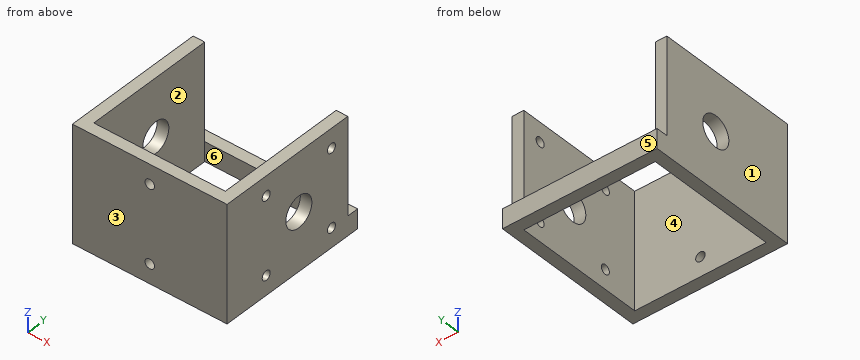
Autodesk Inventor part; units mm, degrees
ref_plane "YZ Plane" through (0, 0, 0) normal (1, 0, 0) x (0, 1, 0)
ref_plane "XZ Plane" through (0, 0, 0) normal (0, 1, 0) x (-1, 0, 0)
ref_plane "XY Plane" through (0, 0, 0) normal (0, 0, 1) x (1, 0, 0)
sketch "スケッチ1" plane through (0, 0, 0) normal (0, 0, 1) x (1, 0, 0)
  line L0 (0, 0) -> (40, 0)
  line L1 (40, 0) -> (40, 40)
  line L2 (40, 40) -> (0, 40)
  line L3 (0, 40) -> (0, 0)
  dimension "d0" = 40
  dimension "d1" = 40
extrude "押し出し1" add sketch "スケッチ1" along normal blind 40
sketch "スケッチ2" plane through (0, 0, 0) normal (0, 0, -1) x (-1, 0, 0)
  point P0 (0, 0)
sketch "スケッチ3" plane through (0, 0, 40) normal (0, 0, 1) x (1, 0, 0)
  line L0 (3, 3) -> (37, 3)
  line L1 (37, 3) -> (37, 37)
  line L2 (37, 37) -> (3, 37)
  line L3 (3, 37) -> (3, 3)
  line L4 (0, 40) -> (0, 0)
  line L5 (40, 40) -> (0, 40)
  line L6 (40, 0) -> (40, 40)
  line L7 (0, 0) -> (40, 0)
  dimension "d4" = 3
  dimension "d5" = 3
  dimension "d6" = 3
  dimension "d7" = 3
extrude "押し出し2" cut sketch "スケッチ3" against normal through all contours L3 L2 L1 L0
sketch "スケッチ4" plane through (0, 40, 0) normal (0, 1, 0) x (1, 0, 0)
  line L0 (0, 0) -> (0, -40)
  line L1 (40, 0) -> (40, -40)
  line L2 (0, -40) -> (40, -40)
  line L3 (40, -40) -> (40, -5)
  line L4 (40, -5) -> (0, -5)
  line L5 (0, -5) -> (0, -40)
  line L6 (40, 0) -> (0, 0)
  point P0 (0, -5)
  dimension "d10" = 5
extrude "押し出し3" cut sketch "スケッチ4" against normal blind 3 contours L4 L1 L2 L0
sketch "スケッチ5" plane through (0, 0, 0) normal (0, -1, 0) x (1, 0, 0)
  line L0 (0, 40) -> (0, 5)
  line L1 (0, 30) -> (40, 30)
  line L2 (40, 5) -> (40, 40)
  line L3 (0, 40) -> (40, 40)
  point P0 (0, 0)
  dimension "d13" = 10
extrude "押し出し4" cut sketch "スケッチ5" against normal through all
sketch "スケッチ6" plane through (0, 37, 0) normal (0, 1, 0) x (1, 0, 0)
  point P0 (0, 0)
sketch "スケッチ7" plane through (0, 0, 0) normal (0, -1, 0) x (1, 0, 0)
  line L0 (40, 30) -> (0, 30)
  line L1 (0, 0) -> (40, 0)
  line L2 (40, 0) -> (40, 30)
  point P0 (20, 5)
  point P1 (20, 25)
  dimension "d16" = 5
  dimension "d17" = 5
  dimension "d18" = 20
  dimension "d19" = 20
hole "穴1" at (20, 0, 5) at (20, 0, 25) direction (0, 1, 0) diameter 2.459 depth 3
sketch "スケッチ8" plane through (40, 0, 0) normal (1, 0, 0) x (0, 0, -1)
  line L0 (-30, 37) -> (-30, 0)
  line L1 (-5, 37) -> (-30, 37)
  line L2 (0, 0) -> (-30, 0)
  line L3 (0, 0) -> (0, 40)
  line L4 (0, 40) -> (-5, 40)
  point P0 (-25, 32)
  point P1 (-5, 32)
  point P2 (-5, 12)
  point P3 (-25, 12)
  dimension "d27" = 5
  dimension "d28" = 5
  dimension "d29" = 5
  dimension "d30" = 12
  dimension "d31" = 12
  dimension "d32" = 5
  dimension "d33" = 5
  dimension "d34" = 8
hole "穴2" at (40, 32, 25) at (40, 32, 5) at (40, 12, 25) at (40, 12, 5) direction (-1, 0, 0) diameter 2.459 depth 3
sketch "スケッチ9" plane through (40, 0, 0) normal (1, 0, 0) x (0, 0, -1)
  line L0 (-30, 37) -> (-30, 0)
  line L1 (-5, 37) -> (-30, 37)
  line L2 (0, 0) -> (-30, 0)
  point P0 (-15, 22)
  dimension "d42" = 15
  dimension "d44" = 22
hole "穴3" at (40, 22, 15) direction (-1, 0, 0) diameter 8 end through all
properties part number "3SR02_振子支え"
Can you work these out from the model? Positions are in its coordinate system, mm. Face numbers are marked on the shaded views. A direction names the side the tool comes from. Round coordinates to 2 decimals unless told otherwise and drop trailing zeros. Loops run counter-clockwise (first coordinate to the right, second up) from the corner with the lowest first, then second, coordinate; pieces in that order, holes last. Notation, with made-up numbers: (-22.5, 79.5) - (3.5, 79.5) arc R26 cw to (3.5, 105.5) - close; hole circle Ø10 at (32, 86). An arc over 180 degrees is marked (long way). Write item = value, one per line. Start each with the question number.
(1) If we mould it in two halves opening along X, with no side actions, what happens to the marked faces 1, 2, 3 and 4? For each: released by +X, released by -X, zero draft, split by the parting line, or undercut.
(2) If we section it at C-C (z = 15): Please give me the cut outline in (x, y).
(3) If we section it at A-A (x = 8): Please give me the cut outline in (y, z), and give its area (3 significant figures).
(4) If I drill on probe 1 along X at (y, z) = (17.5, 21.25); probe 2 along Z at (x, y) = (20, 0.6); probe 3 along Y at (x, z) = (34, 5.75), over which ranges is the centre line in solid material (lowest first)? Write a range as [from, to].
(5) If we section it at D-D (x = 20): Please give me the cut outline in (y, z).
(6) If we section it at B-B (y = 32): Please give me the cut outline in (x, z), and give its area (3 significant figures).
(7) For P1, Ø4, axis at x = 9, z = 4.5, coming from the -Y side; P2, Ø3, axis at x = 17.5, z = 17.5, coming from the +Y side; P3, Ø0.9, axis at x = 10, y = 38.5, coming from the +Z side; P4, Ø1.5, axis at x = 1.5, z = 16, coming from the +Y side, each with a flat end and sliding along its axis, tell me the tip position at first contact or that it passes through.
(8) For the marked faces 5 and 6, which set-ups out of +Z, -Z, +X, -X, +Y, -Y let a thin tool reach every point of the face, with its end or its side?
Ans:
q1.face_1 = released by -X
q1.face_2 = undercut
q1.face_3 = zero draft
q1.face_4 = undercut
q2.outline = (0, 0) - (40, 0) - (40, 18) - (37, 18) - (37, 3) - (3, 3) - (3, 18) - (0, 18) - close; (0, 26) - (3, 26) - (3, 37) - (0, 37) - close; (37, 26) - (40, 26) - (40, 37) - (37, 37) - close
q3.outline = (0, 0) - (3, 0) - (3, 30) - (0, 30) - close; (37, 0) - (40, 0) - (40, 5) - (37, 5) - close
q3.area = 105 mm²
q4.probe_1 = [0, 3], [37, 40]
q4.probe_2 = [0, 3.77], [6.23, 23.77], [26.23, 30]
q4.probe_3 = [0, 3]
q5.outline = (0, 0) - (3, 0) - (3, 3.77) - (0, 3.77) - close; (0, 6.23) - (3, 6.23) - (3, 23.77) - (0, 23.77) - close; (0, 26.23) - (3, 26.23) - (3, 30) - (0, 30) - close; (37, 0) - (40, 0) - (40, 5) - (37, 5) - close
q6.outline = (0, 0) - (3, 0) - (3, 30) - (0, 30) - close; (37, 0) - (40, 0) - (40, 3.77) - (37, 3.77) - close; (37, 6.23) - (40, 6.23) - (40, 23.77) - (37, 23.77) - close; (37, 26.23) - (40, 26.23) - (40, 30) - (37, 30) - close
q6.area = 165 mm²
q7.P1 = 0
q7.P2 = 3
q7.P3 = 5
q7.P4 = 37
q8.face_5 = +Z, -Z, +X, -X, +Y
q8.face_6 = +Z, -Z
